For this review, take the finished solid that the model builds, in its own axes (mm). Round coordinates to 2 decimals unless told otherwise and drop trailing zeros. Loops run counter-clockwise (first coordinate to the right, second up) from the corner with the lowest first, then second, coordinate; pieces in that order, holes last. Notation, with made-up numbers: M 25,20.25 L 38,20.25 A21 ccw 38,52.25 Z; hole C 3,-26.75 d8. An arc over 180 degrees is marked long. One line per question, with ' | ' between items. Start each with the question number.
1) For pin 1 Ø1.5 at (y, z) = (5, -126.5) entering from -X, flat-tipped, find the tip position at first contact; note if it passes through.
2) We need section A-A (x = -6). Give the boundary of the cut face in (y, z).
3) We need section C-C (z = -51.5). Give the boundary of the cut face in (x, y).
4) For probe 1 along Z at (x, y) = (-6, 2); probe 2 along Z at (x, y) = (-7.25, 7); probe 3 along X at (y, z) = (2.5, -10), list the stretches that pass through material, from the lowest coordinate up. Write a range as from..to.
5) We need section B-B (y = 5). Give the boundary of the cut face in (x, z), and give its area (3 significant figures).
Autodesk Inventor part; units mm, degrees
ref_plane "YZ Plane" through (0, 0, 0) normal (1, 0, 0) x (0, 1, 0)
ref_plane "XZ Plane" through (0, 0, 0) normal (0, 1, 0) x (-1, 0, 0)
ref_plane "XY Plane" through (0, 0, 0) normal (0, 0, 1) x (1, 0, 0)
sketch "草图1" plane through (0, 0, 0) normal (0, 1, 0) x (-1, 0, 0)
  line L0 (0, 0) -> (12, 0)
  line L1 (12, 0) -> (12, -300)
  line L2 (12, -300) -> (0, -300)
  line L3 (0, -300) -> (0, 0)
  dimension "d0" = 12
  dimension "d1" = 300
extrude "拉伸1" add sketch "草图1" along normal blind 8
sketch "草图2" plane through (-12, 0, 0) normal (0, 0, 1) x (1, 0, 0)
  line L0 (0, 8) -> (0, 5)
  line L1 (0, 0) -> (0, 8)
  circle A0 centre (0, 5) radius 1.5
  line L2 (12, 8) -> (0, 8)
  line L3 (6, 8) -> (6, -1.6041)
  line L4 (12, 8) -> (12, 5)
  line L5 (12, 0) -> (12, 8)
  circle A1 centre (12, 5) radius 1.5
  line L6 (0, 8) -> (12, 8)
  point P0 (12, 6.5)
  point P1 (12, 3.5)
  point P2 (0, 6.5)
  point P3 (0, 3.5)
  dimension "d9" = 3
  dimension "d10" = 3
extrude "拉伸2" cut sketch "草图2" against normal through all contours A0 L1 L0 | L4 L5 A1 picked at (0.7027, 4.2973) picked at (11.121, 5.4613)
sketch "草图3" plane through (0, 8, 0) normal (0, 1, 0) x (1, 0, 0)
  line L0 (-12, 0) -> (0, 0)
  line L1 (-6, 0) -> (-6, 10)
  circle A0 centre (-6, 10) radius 2
  line L2 (0, 300) -> (-12, 300)
  line L3 (-6, 300) -> (-6, 290)
  circle A1 centre (-6, 290) radius 2
  dimension "d11" = 10
  dimension "d12" = 4
  dimension "d13" = 10
  dimension "d14" = 4
extrude "拉伸3" cut sketch "草图3" against normal through all
equation "\"折弯半径\" = 厚度"
equation "\"折弯释压宽度\" = 厚度"
equation "\"折弯释压深度\" = 0.5 * 厚度"
equation "\"拐角释压尺寸\" = 4 * 厚度"
equation "\"最小余量\" = 2 * 厚度"
equation "\"过渡半径\" = 折弯半径"
equation "\"Jacobi半径尺寸\" = 折弯半径"
equation "\"间隙大小\" = 厚度"
properties part number "滑轨"
Answers below:
1) pin 1: x = -10.7
2) outline: M 0,-300 L 8,-300 L 8,-292 L 0,-292 Z; M 0,-288 L 8,-288 L 8,-12 L 0,-12 Z; M 0,-8 L 8,-8 L 8,0 L 0,0 Z
3) outline: M -12,0 L 0,0 L 0,3.5 A1.5 cw 0,6.5 L 0,8 L -12,8 L -12,6.5 A1.5 cw -12,3.5 Z
4) probe 1: -300..-292, -288..-12, -8..0 | probe 2: -300..-291.56, -288.44..-11.56, -8.44..0 | probe 3: -12..-8, -4..0
5) outline: M -10.5,-300 L -1.5,-300 L -1.5,0 L -10.5,0 Z; hole C -6,-290 d4; hole C -6,-10 d4 | area: 2,670 mm^2
